Here's how the part is built. I have some questions about the finished solid (model axes, mm). A direction names the side the tool comes from. Give positions to 0.01 mm unless a question says otherwise; leave off trailing zeros. Loops run counter-clockwise (first coordinate to the right, second up) from the corner with the lowest first, then second, coordinate; pieces in that order, holes last. Notation, with made-up numbers: (-39, -20) - (-5, -20) arc R12 ccw to (-5, -16) - close; hole circle Ø1 at (2.25, 26.25). An arc over 180 degrees is marked (long way). Use one line per item in the form item = value.
from build123d import *

# Parameters (mm, degrees)
BOSS_EXTRUDE1_DEPTH = 10


with BuildPart() as part:
    # Sketch1 → Boss-Extrude1 (new body)
    with BuildSketch(Plane.XY):
        with BuildLine():
            Line((-5, 0), (-5, -25))
            Line((-5, -25), (-15, -25))
            Line((-15, -25), (-15, 15))
            Line((-15, 15), (15, 15))
            Line((15, 15), (15, -25))
            Line((15, -25), (5, -25))
            Line((5, -25), (5, 0))
            ThreePointArc((5, 0), (0, 5), (-5, 0))
        make_face()
    extrude(amount=BOSS_EXTRUDE1_DEPTH)


solid = part.part
(1) If we section it at A-A (y = -11): List the corners of the cut face in (x, z) for me, plus the area to 3 significant figures.
Geometry says:
outline = (-15, 0) - (-5, 0) - (-5, 10) - (-15, 10) - close; (5, 0) - (15, 0) - (15, 10) - (5, 10) - close
area = 200 mm²
(2) For P1, Ø4, axis at x = 2, z = 8, coming from the -Y side; P2, Ø2, axis at x = -3.5, z = 1.5, coming from the -Y side; P3, Ø1.5, axis at x = -2, z = 1.5, coming from the -Y side, each with a flat end and sliding along its axis, tell me the tip position at first contact or that it passes through.
Geometry says:
P1 = 3
P2 = 2.18
P3 = 4.18
(3) If we section it at C-C (x = 0): List the corners of the cut face in (y, z) for me, plus the area to 3 significant figures.
Geometry says:
outline = (5, 0) - (15, 0) - (15, 10) - (5, 10) - close
area = 100 mm²
(4) If we section it at B-B (z = 7.75): List the corners of the cut face in (x, y) for me.
Geometry says:
outline = (-15, -25) - (-5, -25) - (-5, 0) arc R5 cw to (5, 0) - (5, -25) - (15, -25) - (15, 15) - (-15, 15) - close
(5) Thinking about a two-plate mould opening in X: for faces 3 (the cylindrical face through (0, 5, 5)), 4 (the flat face through (15, -5, 5)), 5 (the flat face through (10, -25, 5)), 6 (the flat face through (-5, -12, 5)), which applies, pulls with the +X half, pulls with the -X half, needs draft (parallel to the pull), parting line crosses it, or undercut?
Geometry says:
face_3 = undercut
face_4 = pulls with the +X half
face_5 = needs draft
face_6 = undercut
(6) If I drill on probe 1 along X at (y, z) = (-20, 6.75); probe 2 along X at (y, z) = (3, 5.75); probe 3 along Y at (x, z) = (-3.25, 5), over which ranges is the centre line in solid material (lowest first)?
Geometry says:
probe_1 = -15 to -5, 5 to 15
probe_2 = -15 to -4, 4 to 15
probe_3 = 3.8 to 15
(7) If we section it at D-D (x = 4): List the corners of the cut face in (y, z) for me.
Geometry says:
outline = (3, 0) - (15, 0) - (15, 10) - (3, 10) - close
(8) For faces 1 (the flat face through (7, -5, 0)), 2 (the flat face through (5, -13, 5)), which set-ups out of +Z, -Z, +X, -X, +Y, -Y let a thin tool reach every point of the face, with its end or its side?
Geometry says:
face_1 = -Z, +X, -X, +Y, -Y
face_2 = +Z, -Z, -Y
